Part model, mm, in its own coordinate system. Face numbers are marked on the shaded views. A direction names the side the tool comes from. Give positions to 0.01 mm unless a question says otherwise; leave off trailing zeros. Answer as CSV lines item,"result". Start each with the question number.
Item 1: Two-plate mould, pull along Y, no slides. Class the marked faces 1, 2 and 3: +Y half, -Y half, draft (parallel to the pull), parting line (faces both ways), or undercut.
Item 2: 3-axis set-ups, long thin cutter, end or side, ignore diameter. For the marked faces 4 and 5: which of +Z, -Z, +X, -X, +Y, -Y reach the whole face in a straight line?
Item 3: Band-saw the part on B-B, the plane y = 0. Count the separate pieces of the cut face and the enclosed holes in it, then the cut area to 3 significant figures.
Item 4: Pin check, flat tips, straight feed: pin 1 (2 mm diameter, centred on x = 0, y = -9.525, fed in from -Z); pin 2 (2 mm diameter, centred on y = 13.5, z = 5, fed in from +X); pin 3 (1.1 mm diameter, centred on y = 0, z = 19.05, fed in from -X); pin 4 (14.5 mm diameter, centred on x = -6.5, y = 6, fed in from -Z). Stop position of each tip, or through.
Item 5: Wall check: L1, parallel to Y at x = 0, z = 23; L2, parallel to X at y = -4, z = 7; L3, parallel to X at y = 0.5, z = 8.5. Give the ranges that are in metal, low to high. Write a range as from..to.
from build123d import *

# Parameters (mm, degrees)
SKETCH1_R                   = 25.4
BOSS_EXTRUDE1_DEPTH         = 38.1
BOSS_EXTRUDE1_DEPTH_BACK    = 44.45
SKETCH2_OUTSIDE_W           = 74.686
SKETCH2_OUTSIDE_H           = 74.686
SKETCH2_OUTSIDE_R           = 17.4625
CUT_EXTRUDE3_DEPTH          = 63.5
SKETCH3_R                   = 23.495
BOSS_EXTRUDE2_DEPTH         = 3.175
F_1_4_28_TAPPED_HOLE1_D     = 5.4102
F_1_4_28_TAPPED_HOLE1_DEPTH = 12.88034
F_1_4_28_TAPPED_HOLE1_TIP   = 1.625388061
SKETCH9_R                   = 0.8636
CUT_EXTRUDE4_DEPTH          = 91.02678768
SKETCH12_R                  = 4.953
CUT_EXTRUDE5_DEPTH          = 45.72
SKETCH17_R                  = 1.651
CUT_EXTRUDE7_DEPTH          = 44.45
SKETCH22_OUTSIDE_W          = 74.686
SKETCH22_OUTSIDE_H          = 74.686
SKETCH22_OUTSIDE_R          = 7.9375
CUT_EXTRUDE9_DEPTH          = 19.05
CHAMFER1_SIZE               = 3.175
F_2_56_TAPPED_HOLE3_REACH   = 81.131
F_2_56_TAPPED_HOLE3_BORE_R  = 0.889
F_2_56_TAPPED_HOLE4_REACH   = 81.131
F_2_56_TAPPED_HOLE4_BORE_R  = 0.889
CIRPATTERN1_COUNT           = 3
SKETCH25_OUTSIDE_W          = 70.184
SKETCH25_OUTSIDE_H          = 70.184
SKETCH25_OUTSIDE_R          = 15.875
CUT_EXTRUDE10_DEPTH         = 25.4


with BuildPart() as part:
    # Sketch1 → Boss-Extrude1 (new, two sides)
    with BuildSketch(Plane.XY) as boss_extrude1_sk:
        Circle(SKETCH1_R)
    extrude(amount=BOSS_EXTRUDE1_DEPTH)
    extrude(boss_extrude1_sk.sketch, amount=-BOSS_EXTRUDE1_DEPTH_BACK)

    # Sketch2 outside → Cut-Extrude3 (cut)
    with BuildSketch(Plane.XY.offset(38.1)):
        Rectangle(SKETCH2_OUTSIDE_W, SKETCH2_OUTSIDE_H)
        Circle(SKETCH2_OUTSIDE_R, mode=Mode.SUBTRACT)
    extrude(amount=-CUT_EXTRUDE3_DEPTH, mode=Mode.SUBTRACT)

    # Sketch3 → Boss-Extrude2 (add)
    with BuildSketch(Plane.XY):
        Circle(SKETCH3_R)
    extrude(amount=BOSS_EXTRUDE2_DEPTH)

    # 1/4-28 Tapped Hole1
    with Locations(Plane.XY.offset(38.1)):
        with Locations((0, 0)):
            Hole(F_1_4_28_TAPPED_HOLE1_D / 2, depth=F_1_4_28_TAPPED_HOLE1_DEPTH)
            with Locations((0, 0, -(F_1_4_28_TAPPED_HOLE1_DEPTH + F_1_4_28_TAPPED_HOLE1_TIP / 2))):  # 118° drill point
                Cone(0, F_1_4_28_TAPPED_HOLE1_D / 2, F_1_4_28_TAPPED_HOLE1_TIP, mode=Mode.SUBTRACT)

    # Sketch6 → #2 Clearance Hole1 (revolve, cut)
    with BuildSketch(Plane(origin=(0, 20.955, 3.175), x_dir=(0, -1, 0), z_dir=(1, 0, 0))):
        Polygon((0, 0), (0, 13.559492758), (1.1303, 12.88034), (1.1303, 0), align=None)
    f_2_clearance_hole1 = revolve(axis=Axis((0, 20.955, 9.525), (0, 0, -1)), mode=Mode.SUBTRACT)

    # Sketch9 → Cut-Extrude4 (cut, through all)
    with BuildSketch(Plane(origin=(0, 0, -44.45), x_dir=(-1, 0, 0), z_dir=(0, 0, -1))):
        Circle(SKETCH9_R)
    extrude(amount=-CUT_EXTRUDE4_DEPTH, mode=Mode.SUBTRACT)

    # Sketch12 → Cut-Extrude5 (cut)
    with BuildSketch(Plane.XY.offset(38.1)):
        with Locations((-10.16, 0)):
            Circle(SKETCH12_R)
        with Locations((10.16, 0)):
            Circle(SKETCH12_R)
    extrude(amount=-CUT_EXTRUDE5_DEPTH, mode=Mode.SUBTRACT)

    # Sketch17 → Cut-Extrude7 (cut)
    with BuildSketch(Plane.XY.offset(38.1)):
        with Locations((0, -9.525)):
            Circle(SKETCH17_R)
    extrude(amount=-CUT_EXTRUDE7_DEPTH, mode=Mode.SUBTRACT)

    # Sketch22 outside → Cut-Extrude9 (cut)
    with BuildSketch(Plane(origin=(0, 0, -44.45), x_dir=(-1, 0, 0), z_dir=(0, 0, -1))):
        Rectangle(SKETCH22_OUTSIDE_W, SKETCH22_OUTSIDE_H)
        Circle(SKETCH22_OUTSIDE_R, mode=Mode.SUBTRACT)
    extrude(amount=-CUT_EXTRUDE9_DEPTH, mode=Mode.SUBTRACT)

    # Chamfer1
    chamfer1_edges = [part.edges().sort_by_distance(p)[0] for p in [
        (-17.4625, 0, -25.4),
        (7.9375, 0, -44.45),
    ]]
    chamfer(chamfer1_edges, length=CHAMFER1_SIZE)

    # #2-56 Tapped Hole3 bore (on position points) → #2-56 Tapped Hole3 (cut, up to next)
    with BuildSketch(Plane(origin=(0, -17.4625, 19.05), x_dir=(-1, 0, 0), z_dir=(0, -1, 0)), mode=Mode.PRIVATE) as f_2_56_tapped_hole3_sk1:
        Circle(F_2_56_TAPPED_HOLE3_BORE_R)
    f_2_56_tapped_hole3_tool1 = extrude(f_2_56_tapped_hole3_sk1.sketch, amount=-F_2_56_TAPPED_HOLE3_REACH, mode=Mode.PRIVATE) & part.part
    add(f_2_56_tapped_hole3_tool1.solids().sort_by_distance((0, -17.4625, 19.05))[0], mode=Mode.SUBTRACT)

    # #2-56 Tapped Hole4 bore (on position points) → #2-56 Tapped Hole4 (cut, up to next)
    with BuildSketch(Plane(origin=(17.4625, 0, 19.05), x_dir=(0, 0, 1), z_dir=(1, 0, 0)), mode=Mode.PRIVATE) as f_2_56_tapped_hole4_sk1:
        Circle(F_2_56_TAPPED_HOLE4_BORE_R)
    f_2_56_tapped_hole4_tool1 = extrude(f_2_56_tapped_hole4_sk1.sketch, amount=-F_2_56_TAPPED_HOLE4_REACH, mode=Mode.PRIVATE) & part.part
    f_2_56_tapped_hole4 = f_2_56_tapped_hole4_tool1.solids().sort_by_distance((17.4625, 0, 19.05))[0]
    add(f_2_56_tapped_hole4, mode=Mode.SUBTRACT)

    # Mirror2: #2-56 Tapped Hole4 across plane
    add(f_2_56_tapped_hole4.mirror(Plane(origin=(0, 0, 0), x_dir=(0, 0, 1), z_dir=(1, 0, 0))), mode=Mode.SUBTRACT)

    # CirPattern1: #2 Clearance Hole1 ×3 about axis
    cirpattern1_axis = Axis((0, 0, 0), (0, 0, 1))
    for i in range(1, CIRPATTERN1_COUNT):
        add(f_2_clearance_hole1.rotate(cirpattern1_axis, i * 360 / CIRPATTERN1_COUNT), mode=Mode.SUBTRACT)

    # Sketch25 outside → Cut-Extrude10 (cut)
    with BuildSketch(Plane(origin=(0, 0, -25.4), x_dir=(-1, 0, 0), z_dir=(0, 0, -1))):
        Rectangle(SKETCH25_OUTSIDE_W, SKETCH25_OUTSIDE_H)
        Circle(SKETCH25_OUTSIDE_R, mode=Mode.SUBTRACT)
    extrude(amount=-CUT_EXTRUDE10_DEPTH, mode=Mode.SUBTRACT)


solid = part.part
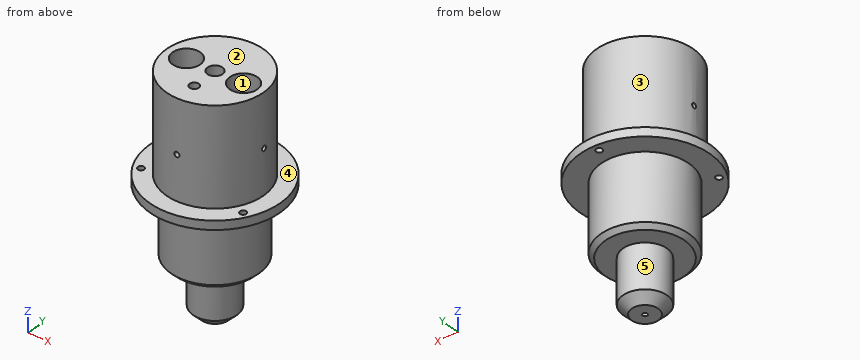
Output:
1,face 1,"undercut"
1,face 2,"draft"
1,face 3,"parting line"
2,face 4,"+Z"
2,face 5,"-Z"
3,separate pieces,"4"
3,enclosed holes,"0"
3,area,"1,360 mm²"
4,pin 1,"z = -25.4"
4,pin 2,"x = 12.19"
4,pin 3,"x = -5.24"
4,pin 4,"z = -44.45"
5,L1,"-17.46..-11.18, -7.87..-0.86, 0.86..17.46"
5,L2,"-17..-13.08, -7.24..7.24, 13.08..17"
5,L3,"-17.46..-15.09, -5.23..-0.7, 0.7..5.23, 15.09..17.46"
